Geometry check sheet. Reference: drawing and pictorial views, mm from the part's lowest x, y, z. A direction names the side the tool comes from. Round coordinates to 2 decimals unless told otherwise and drop trailing zeros. Loops run counter-clockwise (first coordinate to the right, second up) from the corner with the lowest first, then second, coordinate; pieces in that order, holes last. Notation, with made-up numbers: (-30, 84.5) - (1, 84.5) arc R27 cw to (1, 111.5) - close; hole circle Ø10 at (56, 48). An arc over 180 degrees is marked (long way). Return JSON: item names as keys, results as strings.
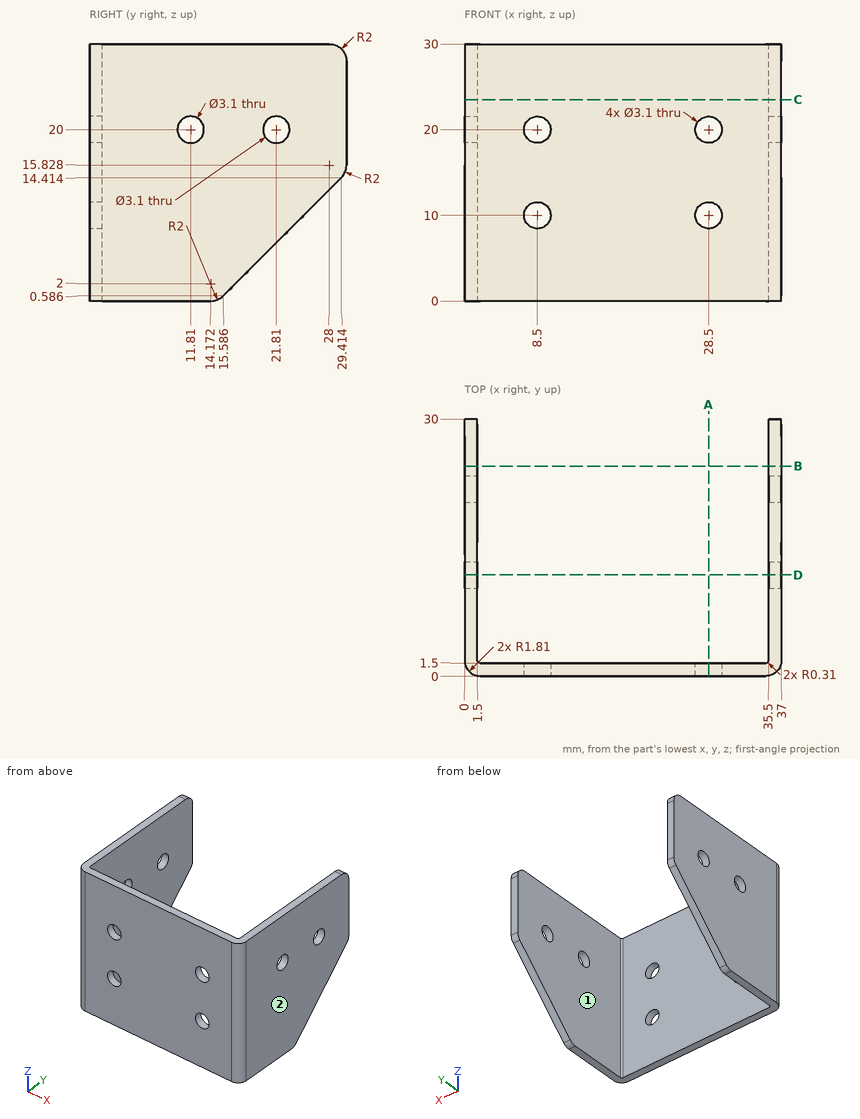
Q1. Sectioned sample at C-C (z = 23.5). Enter the section's corners in (x, y).
Answer key:
{"outline": "(0, 1.81) arc R1.81 ccw to (1.81, 0) - (35.19, 0) arc R1.81 ccw to (37, 1.81) - (37, 30) - (35.5, 30) - (35.5, 1.81) arc R0.31 cw to (35.19, 1.5) - (1.81, 1.5) arc R0.31 cw to (1.5, 1.81) - (1.5, 30) - (0, 30) - close"}
Q2. Sectioned sample at D-D (y = 11.81). Enter the section's corners in (x, z).
Answer key:
{"outline": "(0, 0) - (1.5, 0) - (1.5, 18.45) - (0, 18.45) - close; (0, 21.55) - (1.5, 21.55) - (1.5, 30) - (0, 30) - close; (35.5, 0) - (37, 0) - (37, 18.45) - (35.5, 18.45) - close; (35.5, 21.55) - (37, 21.55) - (37, 30) - (35.5, 30) - close"}
Q3. Tool access check on the marked faces 1 and 2. Record the directions out of +Z, -Z, +X, -X, +Y, -Y that give a thin tool (end or side, any length) a straight path to the whole face; none if there is none.
Answer key:
{"face 1": "+Z, -Z, +Y", "face 2": "+Z, -Z, +X, +Y, -Y"}
Q4. Scan lines: probe 1 along X at (y, z) = (28, 19.75); probe 2 along Y at (x, z) = (36.4, 20) (1 decimal); probe 3 along Y at (x, z) = (31.5, 21.75). Record each from-to range of solid material in increasing order. Write a range as [from, to].
Answer key:
{"probe 1": "x = [0, 1.5], [35.5, 37]", "probe 2": "y = [0.5, 10.3], [13.4, 20.3], [23.4, 30]", "probe 3": "y = [0, 1.5]"}
Q5. Depth check by flat-ended pin: P1, Ø9, axis at x = 19.5, z = 8, coming from the +Y side; P2, Ø3, axis at x = 8.5, z = 10, coming from the -Y side. Enter the tip coordinate at first touch or a pass-through.
Answer key:
{"P1": "stops at y = 1.5", "P2": "passes through"}
Q6. Sectioned sample at A-A (x = 28.5). Enter the section's corners in (y, z).
Answer key:
{"outline": "(0, 0) - (1.5, 0) - (1.5, 8.45) - (0, 8.45) - close; (0, 11.55) - (1.5, 11.55) - (1.5, 18.45) - (0, 18.45) - close; (0, 21.55) - (1.5, 21.55) - (1.5, 30) - (0, 30) - close"}
Q7. Sectioned sample at B-B (y = 24.5). Enter the section's corners in (x, z).
Answer key:
{"outline": "(0, 9.5) - (1.5, 9.5) - (1.5, 30) - (0, 30) - close; (35.5, 9.5) - (37, 9.5) - (37, 30) - (35.5, 30) - close"}
